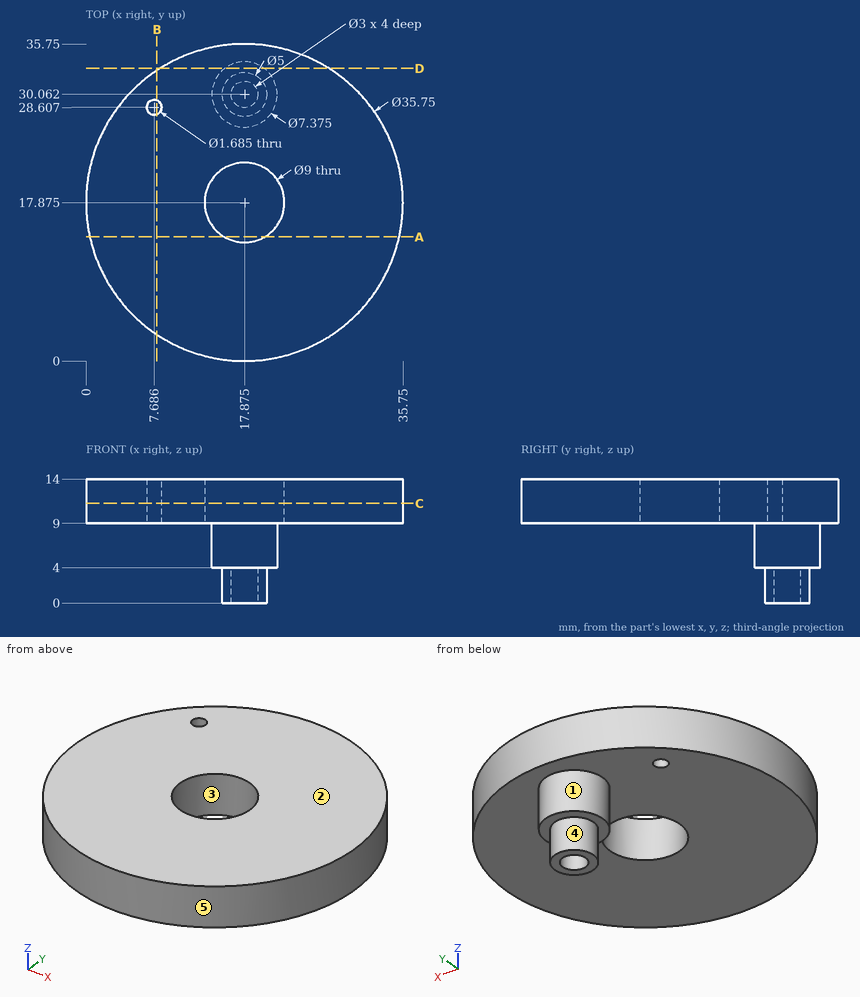
Verification items for this drawing (mm, ordinates from the low corner). A direction names the side the tool comes from. Coordinates: 2 decimals unless noted, no trailing zeros. Order: outer loops, then holes, each group sorted by start corner. A loop starts at its lowest first (then second) coordinate and runs counter-clockwise, first axis right, second up. Notation, with made-up numbers: (2, 74.5) -> (50, 74.5) arc R14 cw to (50, 93.5) -> close; hole circle Ø4 at (52, 71.25). An arc over 180 degrees is marked (long way). Answer as CSV lines item,"result". Start each with the question number.
1) Cross-section at B-B, the plane x = 8. Record the boundary of the cut face in (y, z) (1 decimal).
2) Material ranges on L1, parallel to Z at x = 27, y = 24; L2, parallel to Y at x = 8, z = 13.25 (1 decimal); L3, parallel to X at y = 29, z = 7 (1 decimal), recorded low to high. Write a range as [from, to].
3) Set-up check for the marked faces 4 and 5: record each of +Z, -Z, +X, -X, +Y, -Y from which the full face is reachable in a straight line by a thin tool's end or side.
4) Cross-section at A-A, the plane y = 14. Record the boundary of the cut face in (x, z) (1 decimal), then the cut area to 3 significant figures.
5) Gauge pin test, flat ends, axial feed: pin 1 Ø1.8 at (x, y) = (17.88, 30.06) entering from -Z; pin 2 Ø6 at (y, z) = (27, 7.5) entering from +X (1 decimal); pin 3 Ø12 at (x, y) = (9, 16.5) entering from -Z. Record the tip position at first contact, or that the pin passes through.
6) Cross-section at D-D, the plane y = 33. Record the boundary of the cut face in (x, z) (1 decimal).
7) Release check for a two-part mould opening along X. For the marked faces 1, 2 and 3 record: released by +X, released by -X, zero draft, split by the parting line, or undercut.
8) Cross-section at C-C, the plane z = 11.25. Give the number of separate pieces and of enclosed holes in the cut face, then the cut area to 3 significant figures.
Conclusion:
1,outline,"(3, 9) -> (27.8, 9) -> (27.8, 14) -> (3, 14) -> close; (29.4, 9) -> (32.8, 9) -> (32.8, 14) -> (29.4, 14) -> close"
2,L1,"z = [9, 14]"
2,L2,"y = [3, 27.8], [29.4, 32.8]"
2,L3,"x = [14.3, 21.4]"
3,face 4,"-Z"
3,face 5,"+Z, -Z"
4,outline,"(0.4, 9) -> (15.6, 9) -> (15.6, 14) -> (0.4, 14) -> close; (20.2, 9) -> (35.3, 9) -> (35.3, 14) -> (20.2, 14) -> close"
4,area,"152 mm²"
5,pin 1,"stops at z = 4"
5,pin 2,"stops at x = 34.5"
5,pin 3,"stops at z = 9"
6,outline,"(8.3, 9) -> (15.6, 9) -> (15.6, 4) -> (20.1, 4) -> (20.1, 9) -> (27.4, 9) -> (27.4, 14) -> (8.3, 14) -> close"
7,face 1,"split by the parting line"
7,face 2,"zero draft"
7,face 3,"undercut"
8,separate pieces,"1"
8,enclosed holes,"2"
8,area,"938 mm²"
